```python
from build123d import *

# Parameters (mm, degrees)
SALIENTE_EXTRUIR1_DEPTH = 0.5
SALIENTE_EXTRUIR2_DEPTH = 14


with BuildPart() as part:
    # Croquis1 → Saliente-Extruir1 (new body)
    with BuildSketch(Plane(origin=(0, 0, 0), x_dir=(1, 0, 0), z_dir=(0, 1, 0))):
        Polygon((0, 0), (14, 0), (14, 14), (25, 14), (25, 18.66), (14, 18.66), (14, 30.34), (25, 30.34), (25, 35), (14, 35), (14, 49), (0, 49), align=None)
    extrude(amount=SALIENTE_EXTRUIR1_DEPTH)

    # Croquis2 → Saliente-Extruir2 (add, through all)
    with BuildSketch(Plane(origin=(14, 0, 0), x_dir=(0, 0, -1), z_dir=(1, 0, 0))):
        Polygon((0, 0.5), (-0.5, 0.5), (-0.5, -11.5), (0, -11.5), (0, 0), align=None)
        Polygon((49.5, 0.5), (49.5, -11.5), (49, -11.5), (49, 0), (49, 0.5), align=None)
    extrude(amount=-SALIENTE_EXTRUIR2_DEPTH)


solid = part.part
```
Geometry: final body of the model. Coordinates: model frame, mm. A direction names the side the tool comes from. Coordinates: 2 decimals unless noted, no trailing zeros. Write each loop counter-clockwise with the first axis right and the second up, starting at its lowest first coordinate (ties: lowest second). Pieces come first, ordered by that corner, then holes. Notation, with made-up numbers: M 11.5,-27.75 L 22.5,-27.75 A20 cw 22.5,-23.75 Z; hole C 25,69.25 d1. An arc over 180 degrees is marked long. Answer as CSV lines item,"result". Start each with the question number.
Q1. Mould query, pull axis Z, two halves, no side actions, for faces 4 (the flat face through (7, -5, 0.5)), 5 (the flat face through (14, 0.2, -45.4)), 6 (the flat face through (7, -6, 0)). Classes: released by +Z, released by -Z, zero draft, split by the parting line, or undercut.
Q2. Pin query (flat end, axial travel): P1, Ø7.5, axis at x = 14.5, z = -31, coming from the -Y side; P2, Ø0.6, axis at x = 19.5, y = 0.5, coming from the -Z side. Return the tip coordinate at first contact, or that it passes through.
Q3. Reachability of faces 1 (the flat face through (7, -5, -49.5)), 2 (the flat face through (7, -6, -49)), 3 (the flat face through (14, 0.3, -3.5)) from +Z, -Z, +X, -X, +Y, -Y: full face, straight path, thin tool, end or side. Return the list, or none.
Q4. Cut plane D-D on z = -38.5. Return the cut outline in (x, y).
Q5. Cut plane C-C on x = 13.5. Return the cut outline in (y, z), then the cut area to 3 significant figures.
Q6. Cut plane B-B on x = 17.5. Return the cut outline in (y, z), then the cut area to 3 significant figures.
Q7. Cut plane A-A on y = -4.75. Return the cut outline in (x, z), then the cut area to 3 significant figures.
Q8. Line query: line 1 (Z direction, x = 4.25, y = -2); line 2 (Y direction, x = 2.75, z = -17.5). Output: solid intervals per line, ascending. Write a range as from..to.
Findings below:
1,face 4,"released by +Z"
1,face 5,"zero draft"
1,face 6,"undercut"
2,P1,"stops at y = 0"
2,P2,"stops at z = -35"
3,face 1,"-Z, +X, -X, +Y, -Y"
3,face 2,"+X, -X, -Y"
3,face 3,"+Z, +X, +Y, -Y"
4,outline,"M 0,0 L 14,0 L 14,0.5 L 0,0.5 Z"
5,outline,"M -11.5,-49.5 L 0.5,-49.5 L 0.5,0.5 L -11.5,0.5 L -11.5,0 L 0,0 L 0,-49 L -11.5,-49 Z"
5,area,"36.5 mm2"
6,outline,"M 0,-35 L 0.5,-35 L 0.5,-30.34 L 0,-30.34 Z; M 0,-18.66 L 0.5,-18.66 L 0.5,-14 L 0,-14 Z"
6,area,"4.66 mm2"
7,outline,"M 0,-49.5 L 14,-49.5 L 14,-49 L 0,-49 Z; M 0,0 L 14,0 L 14,0.5 L 0,0.5 Z"
7,area,"14.0 mm2"
8,line 1,"z = -49.5..-49, 0..0.5"
8,line 2,"y = 0..0.5"
